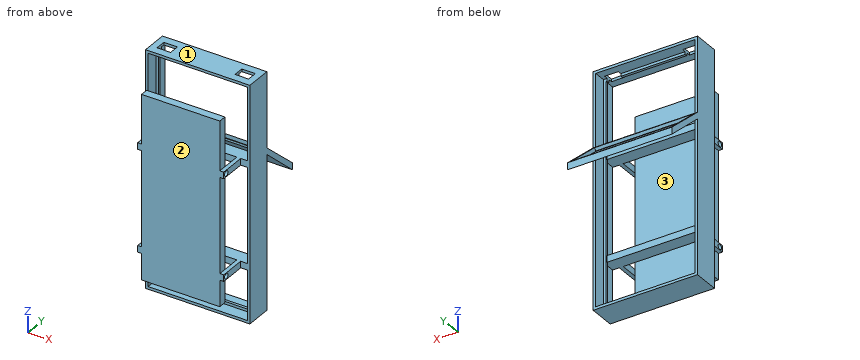
from build123d import *

# Parameters (mm, degrees)
SKETCH1_W            = 101.6
SKETCH1_H            = 50.8
BOSS_EXTRUDE1_DEPTH  = 228.6
SKETCH2_W            = 96.52
SKETCH2_H            = 172.72
CUT_EXTRUDE1_DEPTH   = 50.8
BOSS_EXTRUDE2_DEPTH  = 50.8
BOSS_EXTRUDE3_DEPTH  = 101.6
SKETCH13_W           = 96.52
SKETCH13_H           = 25.4
CUT_EXTRUDE2_DEPTH   = 50.8
SKETCH14_W           = 96.52
SKETCH14_H           = 25.4
CUT_EXTRUDE3_DEPTH   = 50.8
SKETCH15_W           = 96.52
SKETCH15_H           = 50.8
CUT_EXTRUDE6_DEPTH   = 6.35
SKETCH16_W           = 96.52
SKETCH16_H           = 45.72
CUT_EXTRUDE7_DEPTH   = 3.175
SKETCH17_W           = 101.6
SKETCH17_H           = 25.4
CUT_EXTRUDE8_DEPTH   = 228.6
SKETCH19_W           = 6.35
SKETCH19_H           = 12.7
BOSS_EXTRUDE4_DEPTH  = 96.52
SKETCH20_W           = 6.35
SKETCH20_H           = 12.7
BOSS_EXTRUDE5_DEPTH  = 101.6
SKETCH24_W           = 12.7
SKETCH24_H           = 6.35
BOSS_EXTRUDE8_DEPTH  = 19.05
SKETCH25_W           = 12.7
SKETCH25_H           = 6.35
BOSS_EXTRUDE9_DEPTH  = 19.05
SKETCH26_W           = 12.7
SKETCH26_H           = 6.35
BOSS_EXTRUDE10_DEPTH = 19.05
SKETCH27_W           = 12.7
SKETCH27_H           = 6.35
BOSS_EXTRUDE11_DEPTH = 19.05
SKETCH28_W           = 8.89
SKETCH28_H           = 19.05
CUT_EXTRUDE9_DEPTH   = 6.35
SKETCH29_W           = 8.89
SKETCH29_H           = 19.05
CUT_EXTRUDE10_DEPTH  = 6.35
SKETCH30_W           = 8.89
SKETCH30_H           = 19.05
CUT_EXTRUDE11_DEPTH  = 6.35
SKETCH31_W           = 8.89
SKETCH31_H           = 19.05
CUT_EXTRUDE12_DEPTH  = 6.35
SKETCH33_W           = 96.52
SKETCH33_H           = 2.54
BOSS_EXTRUDE13_DEPTH = 2.54
SKETCH34_W           = 96.52
SKETCH34_H           = 2.54
BOSS_EXTRUDE17_DEPTH = 2.54
SKETCH36_W           = 218.44
SKETCH36_H           = 2.54
BOSS_EXTRUDE18_DEPTH = 2.54
SKETCH37_W           = 218.44
SKETCH37_H           = 2.54
BOSS_EXTRUDE19_DEPTH = 2.54
SKETCH42_W           = 6.35
SKETCH42_H           = 6.35
CUT_EXTRUDE16_DEPTH  = 5.08
SKETCH45_W           = 13.208
SKETCH45_H           = 10.16
CUT_EXTRUDE19_DEPTH  = 6.35
SKETCH50_W           = 6.35
SKETCH50_H           = 6.35
BOSS_EXTRUDE20_DEPTH = 3.81
SKETCH51_W           = 6.35
SKETCH51_H           = 6.35
BOSS_EXTRUDE21_DEPTH = 3.81
SKETCH52_W           = 6.35
SKETCH52_H           = 6.35
BOSS_EXTRUDE22_DEPTH = 3.81
SKETCH53_W           = 6.35
SKETCH53_H           = 6.35
BOSS_EXTRUDE23_DEPTH = 3.81
SKETCH54_W           = 6.35
SKETCH54_H           = 6.35
BOSS_EXTRUDE24_DEPTH = 3.81
SKETCH55_W           = 76.2
SKETCH55_H           = 177.8
BOSS_EXTRUDE25_DEPTH = 7.62
SKETCH56_R           = 2.54
CUT_EXTRUDE20_DEPTH  = 83.82
SKETCH57_R           = 2.54
CUT_EXTRUDE21_DEPTH  = 83.82


with BuildPart() as part:
    # Sketch1 → Boss-Extrude1 (new body)
    with BuildSketch(Plane.XY):
        Rectangle(SKETCH1_W, SKETCH1_H)
    extrude(amount=-BOSS_EXTRUDE1_DEPTH)

    # Sketch2 → Cut-Extrude1 (cut)
    with BuildSketch(Plane(origin=(0, 25.4, 0), x_dir=(1, 0, 0), z_dir=(0, 1, 0))):
        with Locations((0, 114.3)):
            Rectangle(SKETCH2_W, SKETCH2_H)
    extrude(amount=-CUT_EXTRUDE1_DEPTH, mode=Mode.SUBTRACT)

    # Sketch3 → Boss-Extrude2 (add)
    with BuildSketch(Plane(origin=(0, 25.4, 0), x_dir=(1, 0, 0), z_dir=(0, 1, 0))):
        Polygon((48.26, 73.001295984), (48.26, 79.351295984), (-48.26, 79.351295984), (-48.26, 73.001295984), (0, 73.001295984), align=None)
    extrude(amount=-BOSS_EXTRUDE2_DEPTH)

    # Sketch11 → Boss-Extrude3 (add)
    with BuildSketch(Plane.ZY.offset(50.8)):
        Polygon((-79.351295984, 25.4), (-113.622558301, 63.5), (-106.756614843, 63.363382999), (-73.001295984, 25.4), align=None)
    extrude(amount=-BOSS_EXTRUDE3_DEPTH)

    # Sketch13 → Cut-Extrude2 (cut)
    with BuildSketch(Plane(origin=(0, 25.4, 0), x_dir=(1, 0, 0), z_dir=(0, 1, 0))):
        with Locations((0, 213.36)):
            Rectangle(SKETCH13_W, SKETCH13_H)
    extrude(amount=-CUT_EXTRUDE2_DEPTH, mode=Mode.SUBTRACT)

    # Sketch14 → Cut-Extrude3 (cut)
    with BuildSketch(Plane(origin=(0, 25.4, 0), x_dir=(1, 0, 0), z_dir=(0, 1, 0))):
        with Locations((0, 15.24)):
            Rectangle(SKETCH14_W, SKETCH14_H)
    extrude(amount=-CUT_EXTRUDE3_DEPTH, mode=Mode.SUBTRACT)

    # Sketch15 → Cut-Extrude6 (cut)
    with BuildSketch(Plane.XY.offset(-73.001295984)):
        Rectangle(SKETCH15_W, SKETCH15_H)
    extrude(amount=-CUT_EXTRUDE6_DEPTH, mode=Mode.SUBTRACT)

    # Sketch16 → Cut-Extrude7 (cut)
    with BuildSketch(Plane(origin=(0, -25.035409247, -28.156416881), x_dir=(1, 0, 0), z_dir=(0, 0.664474781, 0.747310689))):
        with Locations((0, 92.889211639)):
            Rectangle(SKETCH16_W, SKETCH16_H)
    extrude(amount=-CUT_EXTRUDE7_DEPTH, mode=Mode.SUBTRACT)

    # Sketch17 → Cut-Extrude8 (cut)
    with BuildSketch(Plane.XY):
        with Locations((0, -12.7)):
            Rectangle(SKETCH17_W, SKETCH17_H)
    extrude(amount=-CUT_EXTRUDE8_DEPTH, mode=Mode.SUBTRACT)

    # Sketch19 → Boss-Extrude4 (add)
    with BuildSketch(Plane.ZY.offset(-48.26)):
        with Locations((-76.176295984, 6.35)):
            Rectangle(SKETCH19_W, SKETCH19_H)
    extrude(amount=BOSS_EXTRUDE4_DEPTH)

    # Sketch20 → Boss-Extrude5 (add)
    with BuildSketch(Plane.ZY.offset(50.8)):
        with Locations((-174.625, 6.35)):
            Rectangle(SKETCH20_W, SKETCH20_H)
    extrude(amount=-BOSS_EXTRUDE5_DEPTH)

    # Sketch24 → Boss-Extrude8 (add)
    with BuildSketch(Plane.XZ):
        with Locations((44.45, -76.176295984)):
            Rectangle(SKETCH24_W, SKETCH24_H)
    extrude(amount=BOSS_EXTRUDE8_DEPTH)

    # Sketch25 → Boss-Extrude9 (add)
    with BuildSketch(Plane.XZ):
        with Locations((-44.45, -76.176295984)):
            Rectangle(SKETCH25_W, SKETCH25_H)
    extrude(amount=BOSS_EXTRUDE9_DEPTH)

    # Sketch26 → Boss-Extrude10 (add)
    with BuildSketch(Plane.XZ):
        with Locations((-44.45, -174.625)):
            Rectangle(SKETCH26_W, SKETCH26_H)
    extrude(amount=BOSS_EXTRUDE10_DEPTH)

    # Sketch27 → Boss-Extrude11 (add)
    with BuildSketch(Plane.XZ):
        with Locations((44.45, -174.625)):
            Rectangle(SKETCH27_W, SKETCH27_H)
    extrude(amount=BOSS_EXTRUDE11_DEPTH)

    # Sketch28 → Cut-Extrude9 (cut)
    with BuildSketch(Plane.XY.offset(-73.001295984)):
        with Locations((46.355, -9.525)):
            Rectangle(SKETCH28_W, SKETCH28_H)
    extrude(amount=-CUT_EXTRUDE9_DEPTH, mode=Mode.SUBTRACT)

    # Sketch29 → Cut-Extrude10 (cut)
    with BuildSketch(Plane.XY.offset(-73.001295984)):
        with Locations((-46.355, -9.525)):
            Rectangle(SKETCH29_W, SKETCH29_H)
    extrude(amount=-CUT_EXTRUDE10_DEPTH, mode=Mode.SUBTRACT)

    # Sketch30 → Cut-Extrude11 (cut)
    with BuildSketch(Plane.XY.offset(-171.45)):
        with Locations((-46.355, -9.525)):
            Rectangle(SKETCH30_W, SKETCH30_H)
    extrude(amount=-CUT_EXTRUDE11_DEPTH, mode=Mode.SUBTRACT)

    # Sketch31 → Cut-Extrude12 (cut)
    with BuildSketch(Plane.XY.offset(-171.45)):
        with Locations((46.355, -9.525)):
            Rectangle(SKETCH31_W, SKETCH31_H)
    extrude(amount=-CUT_EXTRUDE12_DEPTH, mode=Mode.SUBTRACT)

    # Sketch33 → Boss-Extrude13 (add)
    with BuildSketch(Plane(origin=(0, 0, -2.54), x_dir=(-1, 0, 0), z_dir=(0, 0, -1))):
        with Locations((0, 12.7)):
            Rectangle(SKETCH33_W, SKETCH33_H)
    extrude(amount=BOSS_EXTRUDE13_DEPTH)

    # Sketch34 → Boss-Extrude17 (add)
    with BuildSketch(Plane.XY.offset(-226.06)):
        with Locations((0, 12.7)):
            Rectangle(SKETCH34_W, SKETCH34_H)
    extrude(amount=BOSS_EXTRUDE17_DEPTH)

    # Sketch36 → Boss-Extrude18 (add)
    with BuildSketch(Plane(origin=(-48.26, 0, 0), x_dir=(0, 0, -1), z_dir=(1, 0, 0))):
        with Locations((114.3, 12.7)):
            Rectangle(SKETCH36_W, SKETCH36_H)
    extrude(amount=BOSS_EXTRUDE18_DEPTH)

    # Sketch37 → Boss-Extrude19 (add)
    with BuildSketch(Plane.ZY.offset(-48.26)):
        with Locations((-114.3, 12.7)):
            Rectangle(SKETCH37_W, SKETCH37_H)
    extrude(amount=BOSS_EXTRUDE19_DEPTH)

    # Sketch42 → Cut-Extrude16 (cut)
    with BuildSketch(Plane.ZY.offset(41.91)):
        with Locations((-76.176295984, -15.875)):
            Rectangle(SKETCH42_W, SKETCH42_H)
    extrude(amount=-CUT_EXTRUDE16_DEPTH, mode=Mode.SUBTRACT)

    # Sketch45 → Cut-Extrude19 (cut)
    with BuildSketch(Plane.XY):
        with Locations((37.933039121, 12.7)):
            Rectangle(SKETCH45_W, SKETCH45_H)
        with Locations((-37.933039121, 12.7)):
            Rectangle(SKETCH45_W, SKETCH45_H)
    extrude(amount=-CUT_EXTRUDE19_DEPTH, mode=Mode.SUBTRACT)

    # Sketch50 → Boss-Extrude20 (add)
    with BuildSketch(Plane.ZY.offset(41.91)):
        with Locations((-76.176295984, -15.875)):
            Rectangle(SKETCH50_W, SKETCH50_H)
    extrude(amount=-BOSS_EXTRUDE20_DEPTH)

    # Sketch51 → Boss-Extrude21 (add)
    with BuildSketch(Plane.ZY.offset(41.91)):
        with Locations((-76.176295984, -22.225)):
            Rectangle(SKETCH51_W, SKETCH51_H)
    extrude(amount=-BOSS_EXTRUDE21_DEPTH)

    # Sketch52 → Boss-Extrude22 (add)
    with BuildSketch(Plane.ZY.offset(41.91)):
        with Locations((-174.625, -22.225)):
            Rectangle(SKETCH52_W, SKETCH52_H)
    extrude(amount=-BOSS_EXTRUDE22_DEPTH)

    # Sketch53 → Boss-Extrude23 (add)
    with BuildSketch(Plane(origin=(41.91, 0, 0), x_dir=(0, 0, -1), z_dir=(1, 0, 0))):
        with Locations((76.176295984, -22.225)):
            Rectangle(SKETCH53_W, SKETCH53_H)
    extrude(amount=-BOSS_EXTRUDE23_DEPTH)

    # Sketch54 → Boss-Extrude24 (add)
    with BuildSketch(Plane(origin=(41.91, 0, 0), x_dir=(0, 0, -1), z_dir=(1, 0, 0))):
        with Locations((174.625, -22.225)):
            Rectangle(SKETCH54_W, SKETCH54_H)
    extrude(amount=-BOSS_EXTRUDE24_DEPTH)

    # Sketch55 → Boss-Extrude25 (add)
    with BuildSketch(Plane.XZ.offset(25.4)):
        with Locations((0, -114.3)):
            Rectangle(SKETCH55_W, SKETCH55_H)
    extrude(amount=-BOSS_EXTRUDE25_DEPTH)

    # Sketch56 → Cut-Extrude20 (cut)
    with BuildSketch(Plane.ZY.offset(41.91)):
        with Locations((-76.176295984, -21.59)):
            Circle(SKETCH56_R)
    extrude(amount=-CUT_EXTRUDE20_DEPTH, mode=Mode.SUBTRACT)

    # Sketch57 → Cut-Extrude21 (cut)
    with BuildSketch(Plane.ZY.offset(41.91)):
        with Locations((-174.625, -21.59)):
            Circle(SKETCH57_R)
    extrude(amount=-CUT_EXTRUDE21_DEPTH, mode=Mode.SUBTRACT)


solid = part.part
Here's how the part is built. I have some questions about the finished solid (model axes, mm). Face numbers are marked on the shaded views. Coordinates: 2 decimals unless noted, no trailing zeros. Loops run counter-clockwise (first coordinate to the right, second up) from the corner with the lowest first, then second, coordinate; pieces in that order, holes last.
1. Imagine slicing it at B-B, the plane y = -21.59. Please give me the cut outline in (x, z) (3 decimals).
2. Imagine slicing it at D-D, the plane y = -11. Please give me the cut outline in (x, z).
3. Imagine slicing it at A-A, the plane z = -15. Please give me the cut outline in (x, y), and give its area (3 significant figures).
4. Imagine slicing it at C-C, the plane z = -70.5. Please give me the cut outline in (x, y).
5. I need wall thicknesses on L1, parallel to Z at x = 42, y = 21.5; L2, parallel to X at y = 19.5, z = -151.5; L3, parallel to Y at x = 14.5, z = -68.5. Which ranges of each line are inside material? Lowest first, please.
6. If we mould it in two halves opening along Y, with no side actions, what happens to the marked faces 1, 2 and 3? For each: pulls with the +Y half, pulls with the -Y half, needs draft (parallel to the pull), parting line crosses it, or undercut.
7. For P1, Ø6, axis at y = -20, z = -138, coming from the +X side; P2, Ø1.5, axis at x = 6, z = -84.5, coming from the +Y side; P3, Ø6, axis at x = 0, y = -22.5, coming from the -Z side, each with a flat end and sliding along its axis, tell me the tip position at first contact or that it passes through.
Taken from the geometry:
1. outline: (-41.91, -177.8) - (-38.1, -177.8) - (-38.1, -203.2) - (38.1, -203.2) - (38.1, -177.8) - (41.91, -177.8) - (41.91, -177.165) - (-41.91, -177.165) - close; (-41.91, -172.085) - (41.91, -172.085) - (41.91, -171.45) - (38.1, -171.45) - (38.1, -79.351) - (41.91, -79.351) - (41.91, -78.716) - (-41.91, -78.716) - (-41.91, -79.351) - (-38.1, -79.351) - (-38.1, -171.45) - (-41.91, -171.45) - close; (-41.91, -73.636) - (41.91, -73.636) - (41.91, -73.001) - (38.1, -73.001) - (38.1, -25.4) - (-38.1, -25.4) - (-38.1, -73.001) - (-41.91, -73.001) - close
2. outline: (-41.91, -177.8) - (-38.1, -177.8) - (-38.1, -171.45) - (-41.91, -171.45) - close; (-41.91, -79.35) - (-38.1, -79.35) - (-38.1, -73) - (-41.91, -73) - close; (38.1, -177.8) - (41.91, -177.8) - (41.91, -171.45) - (38.1, -171.45) - close; (38.1, -79.35) - (41.91, -79.35) - (41.91, -73) - (38.1, -73) - close
3. outline: (-50.8, 0) - (-48.26, 0) - (-48.26, 11.43) - (-45.72, 11.43) - (-45.72, 13.97) - (-48.26, 13.97) - (-48.26, 25.4) - (-50.8, 25.4) - close; (45.72, 11.43) - (48.26, 11.43) - (48.26, 0) - (50.8, 0) - (50.8, 25.4) - (48.26, 25.4) - (48.26, 13.97) - (45.72, 13.97) - close
3. area: 142 mm2
4. outline: (-50.8, 0) - (-48.26, 0) - (-48.26, 11.43) - (-45.72, 11.43) - (-45.72, 13.97) - (-48.26, 13.97) - (-48.26, 25.4) - (-50.8, 25.4) - close; (-38.1, -25.4) - (38.1, -25.4) - (38.1, -17.78) - (-38.1, -17.78) - close; (45.72, 11.43) - (48.26, 11.43) - (48.26, 0) - (50.8, 0) - (50.8, 25.4) - (48.26, 25.4) - (48.26, 13.97) - (45.72, 13.97) - close
5. L1: z = -228.6 to -226.06, -2.54 to 0
5. L2: x = -50.8 to -48.26, 48.26 to 50.8
5. L3: y = -25.4 to -17.78
6. face 1: needs draft
6. face 2: pulls with the -Y half
6. face 3: undercut
7. P1: stops at x = 38.1
7. P2: stops at y = 34.4
7. P3: stops at z = -203.2
